Check sheet for the modelled part. Datum: model origin and axes. Units: mm. A direction names the side the tool comes from. Coordinates: 2 decimals unless noted, no trailing zeros. Loops run counter-clockwise (first coordinate to the right, second up) from the corner with the lowest first, then second, coordinate; pieces in that order, holes last. Notation, with made-up numbers: (0, 89.25) -> (14, 89.25) arc R15 cw to (14, 95.25) -> close; hole circle Ø3 at (21, 64.25). An arc over 180 degrees is marked (long way). Use one line per item in the form item = value.
from build123d import *

# Parameters (mm, degrees)
SKETCH_W        = 120
SKETCH_H        = 110
PAD_DEPTH       = 2
SKETCH001_R     = 2.4
POCKET_DEPTH    = 5
SKETCH002_W     = 1.5
SKETCH002_H     = 110
SKETCH002_W_2   = 118.5
SKETCH002_H_2   = 1.5
SKETCH002_H_3   = 108.5
PAD001_DEPTH    = 23
SKETCH003_W     = 10
SKETCH003_H     = 5
POCKET001_DEPTH = 1.5
SKETCH004_W     = 70
SKETCH004_H     = 5
SKETCH004_W_2   = 5
SKETCH004_H_2   = 50
PAD002_DEPTH    = 40
SKETCH005_W     = 75
SKETCH005_H     = 60
PAD003_DEPTH    = 5
SKETCH006_W     = 20
SKETCH006_H     = 7
PAD004_DEPTH    = 11
SKETCH007_W     = 14.1
SKETCH007_H     = 9
POCKET002_DEPTH = 10


with BuildPart() as part:
    # Sketch → Pad (new body)
    with BuildSketch(Plane.XZ):
        with Locations((60, 55)):
            Rectangle(SKETCH_W, SKETCH_H)
    extrude(amount=PAD_DEPTH)

    # Sketch001 (on Face6 of Pad) → Pocket (cut)
    with BuildSketch(Plane.XZ.offset(2)):
        with Locations((12, 19)):
            Circle(SKETCH001_R)
        with Locations((4.5, 77)):
            Circle(SKETCH001_R)
    extrude(amount=-POCKET_DEPTH, mode=Mode.SUBTRACT)

    # Sketch002 (on Face5 of Pocket) → Pad001 (join)
    with BuildSketch(Plane.XZ.offset(2)):
        with Locations((0.75, 55)):
            Rectangle(SKETCH002_W, SKETCH002_H)
        with Locations((60.75, 0.75)):
            Rectangle(SKETCH002_W_2, SKETCH002_H_2)
        with Locations((119.25, 55.75)):
            Rectangle(SKETCH002_W, SKETCH002_H_3)
    extrude(amount=PAD001_DEPTH)

    # Sketch003 (on Face11 of Pad001) → Pocket001 (cut)
    with BuildSketch(Plane(origin=(120, 0, 0), x_dir=(0, 0, 1), z_dir=(1, 0, 0))):
        with Locations((49.672382, 2.5)):
            Rectangle(SKETCH003_W, SKETCH003_H)
    extrude(amount=-POCKET001_DEPTH, mode=Mode.SUBTRACT)

    # Sketch004 (on Face1 of Pocket001) → Pad002 (join)
    with BuildSketch(Plane(origin=(0, 0, 0), x_dir=(1, 0, 0), z_dir=(0, 1, 0))):
        with Locations((60, -32.5)):
            Rectangle(SKETCH004_W, SKETCH004_H)
        with Locations((22.5, -60)):
            Rectangle(SKETCH004_W_2, SKETCH004_H_2)
        with Locations((60, -87.5)):
            Rectangle(SKETCH004_W, SKETCH004_H)
    extrude(amount=PAD002_DEPTH)

    # Sketch005 (on Face30 of Pad002) → Pad003 (join)
    with BuildSketch(Plane(origin=(0, 40, 0), x_dir=(1, 0, 0), z_dir=(0, 1, 0))):
        with Locations((57.5, -60)):
            Rectangle(SKETCH005_W, SKETCH005_H)
    extrude(amount=PAD003_DEPTH)

    # Sketch006 (on Face1 of Pad003) → Pad004 (join)
    with BuildSketch(Plane(origin=(0, 0, 0), x_dir=(1, 0, 0), z_dir=(0, 1, 0))):
        with Locations((60, -106.5)):
            Rectangle(SKETCH006_W, SKETCH006_H)
    extrude(amount=PAD004_DEPTH)

    # Sketch007 (on Face35 of Pad004) → Pocket002 (cut)
    with BuildSketch(Plane(origin=(0, 0, 110), x_dir=(-1, 0, 0), z_dir=(0, 0, 1))):
        with Locations((-60, -5.5)):
            Rectangle(SKETCH007_W, SKETCH007_H)
    extrude(amount=-POCKET002_DEPTH, mode=Mode.SUBTRACT)


solid = part.part
(1) Section check C-C, the plane x = 4.5. Record the boundary of the cut face in (y, z).
Established:
outline = (-25, 0) -> (0, 0) -> (0, 74.6) -> (-2, 74.6) -> (-2, 1.5) -> (-25, 1.5) -> close; (-2, 79.4) -> (0, 79.4) -> (0, 110) -> (-2, 110) -> close
(2) Scan lines: line 1 along Y through (x, z) = (22.5, 33.5); line 2 along Z through (x, y) = (4.5, -1.45); line 3 along Z through (x, y) = (12, -1.3). Record each from-to range of solid material in increasing order.
Established:
line_1 = -2 to 0, 40 to 45
line_2 = 0 to 74.6, 79.4 to 110
line_3 = 0 to 16.6, 21.4 to 110
(3) Tool access check on faces 1 (the flat face through (22, 20, 35)), 2 (the flat face through (20, 22, 60)), 3 (the flat face through (52.95, 6, 107)). Record the directions out of +Z, -Z, +X, -X, +Y, -Y that give a thin tool (end or side, any length) a straight path to the whole face; none if there is none.
Established:
face_1 = -Z, -X
face_2 = +Z, -Z, -X, +Y
face_3 = +Z
(4) Section check B-B, the plane z = 19. Record the boundary of the cut face in (x, y).
Established:
outline = (0, -25) -> (1.5, -25) -> (1.5, -2) -> (9.6, -2) -> (9.6, 0) -> (0, 0) -> close; (14.4, -2) -> (118.5, -2) -> (118.5, -25) -> (120, -25) -> (120, 0) -> (14.4, 0) -> close
(5) Mould release check, pull along Y, two halves, no side actions. Record for faces 4 (the flat face through (120, -12, 54)), 5 (the flat face through (60, 10, 107)), 6 (the flat face through (59, -2, 57)): +Y half, -Y half, draft (parallel to the pull), parting line (faces both ways), or undercut.
Established:
face_4 = draft
face_5 = undercut
face_6 = -Y half
(6) Section check A-A, the plane x = 60.5. Record the boundary of the cut face in (y, z).
Established:
outline = (-25, 0) -> (0, 0) -> (0, 30) -> (45, 30) -> (45, 90) -> (0, 90) -> (0, 103) -> (1, 103) -> (1, 110) -> (-2, 110) -> (-2, 1.5) -> (-25, 1.5) -> close; (10, 103) -> (11, 103) -> (11, 110) -> (10, 110) -> close; hole (0, 35) -> (40, 35) -> (40, 85) -> (0, 85) -> close
(7) Go/stop test with flat-tipped pins: P1, Ø4, axis at y = 25, z = 70.5, coming from the +X side; P2, Ø3, axis at x = 95, z = 78.5, coming from the -Y side; P3, Ø2, axis at y = -1, z = 50, coming from the +X side. Record where each tip stops, or that it passes through.
Established:
P1 = 25
P2 = -2
P3 = 118.5
